from build123d import *

# Parameters (mm, degrees)
BOSS_EXTRUDE1_DEPTH       = 23.1
BOSS_EXTRUDE3_DEPTH       = 1
SKETCH8_R                 = 1.5
BOSS_EXTRUDE4_DEPTH       = 1
M8_TAPPED_HOLE1_D         = 6.8
M8_TAPPED_HOLE1_DEPTH     = 13.75
M8_TAPPED_HOLE1_TIP       = 2.042926105
F_4_0MM_DOWEL_HOLE1_D     = 4
F_4_0MM_DOWEL_HOLE1_DEPTH = 15
F_4_0MM_DOWEL_HOLE1_TIP   = 1.201721238
F_4_0MM_DOWEL_HOLE2_D     = 4
F_4_0MM_DOWEL_HOLE2_DEPTH = 15
F_4_0MM_DOWEL_HOLE2_TIP   = 1.201721238


with BuildPart() as part:
    # Sketch1 → Boss-Extrude1 (new body)
    with BuildSketch(Plane(origin=(0, 0, 0), x_dir=(1, 0, 0), z_dir=(0, 1, 0))):
        with BuildLine():
            Line((0, 7), (25, 7))
            ThreePointArc((25, 7), (32, 0), (25, -7))
            Line((25, -7), (0, -7))
            ThreePointArc((0, -7), (-7, 0), (0, 7))
        make_face()
    extrude(amount=BOSS_EXTRUDE1_DEPTH)

    # Sketch6 → Boss-Extrude3 (add)
    # profile 1 of 3: a face of its own
    with BuildSketch(Plane(origin=(0, 23.1, 0), x_dir=(1, 0, 0), z_dir=(0, 1, 0))):
        with BuildLine():
            Line((1.153846154, 4.5), (2.954927885, 4.5))
            add(Edge.make_bspline(
                [(2.954927885, 4.5), (3.075119358, 4.499599922), (3.305900301, 4.498831727), (3.636517282, 4.494548337), (3.936929817, 4.482271422), (4.206980832, 4.471706493), (4.446665374, 4.452441501), (4.656718407, 4.434028409), (4.836172486, 4.40992471), (4.944804675, 4.387539336), (4.993990385, 4.377403846)],
                knots=[0, 0, 0, 0, 1.410062039, 2.707475311, 3.878576406, 4.937260626, 5.877586885, 6.699081471, 7.410979367, 8, 8, 8, 8], degree=3))
            add(Edge.make_bspline(
                [(4.993990385, 4.377403846), (5.05983599, 4.361135021), (5.190122534, 4.328944429), (5.377708418, 4.260905455), (5.556459537, 4.182169278), (5.725633371, 4.08969114), (5.884382548, 3.982784563), (6.034343919, 3.863295106), (6.176197967, 3.731876576), (6.304207874, 3.585215555), (6.424908292, 3.431350245), (6.526707617, 3.264969156), (6.614461422, 3.090982371), (6.684328466, 2.907620439), (6.740586112, 2.716661597), (6.780253585, 2.51637612), (6.804042353, 2.30767647), (6.806464267, 2.165327562), (6.807692308, 2.093149038)],
                knots=[0, 0, 0, 0, 1.027469482, 2.033020251, 3.019912614, 3.986113645, 4.951240523, 5.91722682, 6.890402269, 7.87763091, 8.8651537, 9.85103654, 10.82876324, 11.815024772, 12.821070561, 13.842952187, 14.906261191, 16, 16, 16, 16], degree=3))
            add(Edge.make_bspline(
                [(6.807692308, 2.093149038), (6.803914884, 1.973230198), (6.796544152, 1.739237481), (6.727822457, 1.399652357), (6.615254263, 1.082879834), (6.460137234, 0.789318765), (6.26260144, 0.524691391), (6.025194834, 0.292258792), (5.747784976, 0.097756159), (5.489538163, -0.037122481), (5.261415936, -0.123504247), (5.073615988, -0.184283455), (4.868758046, -0.231242794), (4.6488049, -0.273311705), (4.412841215, -0.305073204), (4.161432542, -0.328335876), (3.894399581, -0.342874858), (3.710956259, -0.345040014), (3.616586538, -0.346153846)],
                knots=[0, 0, 0, 0, 1.260483769, 2.459530307, 3.627416485, 4.787058657, 5.939039949, 7.08810263, 8.267026773, 9.491475466, 10.141966685, 10.831826277, 11.566392101, 12.351337768, 13.187381173, 14.07005841, 15.007169909, 16, 16, 16, 16], degree=3))
            Line((3.616586538, -0.346153846), (6.923076923, -4.5))
            Line((6.923076923, -4.5), (5.924278846, -4.5))
            Line((5.924278846, -4.5), (2.617788462, -0.346153846))
            Line((2.617788462, -0.346153846), (1.961538462, -0.346153846))
            Line((1.961538462, -0.346153846), (1.961538462, -4.5))
            Line((1.961538462, -4.5), (1.153846154, -4.5))
            Line((1.153846154, -4.5), (1.153846154, 4.5))
        make_face()
        with BuildLine():
            Line((1.961538462, 3.576923077), (1.961538462, 0.576923077))
            Line((1.961538462, 0.576923077), (3.609375, 0.564302885))
            add(Edge.make_bspline(
                [(3.609375, 0.564302885), (3.686312243, 0.564268848), (3.835438533, 0.564202874), (4.051183099, 0.574472584), (4.252063387, 0.586155403), (4.437311035, 0.604025148), (4.6070088, 0.627055047), (4.761071863, 0.655862721), (4.89975171, 0.689425168), (5.061490809, 0.741372205), (5.242099033, 0.823673395), (5.43837993, 0.943413249), (5.605528798, 1.094019555), (5.746746158, 1.266237014), (5.860221839, 1.455587368), (5.940224265, 1.659800889), (5.990990545, 1.873722141), (5.996978233, 2.020751561), (6, 2.094951923)],
                knots=[0, 0, 0, 0, 1.146690395, 2.22261258, 3.21895312, 4.145990853, 4.996080663, 5.770904154, 6.481378293, 7.121626537, 8.300444488, 9.431385265, 10.535395872, 11.636531494, 12.74115979, 13.810798291, 14.895190096, 16, 16, 16, 16], degree=3))
            add(Edge.make_bspline(
                [(6, 2.094951923), (5.996908831, 2.167328827), (5.990783263, 2.310753441), (5.940772144, 2.520725781), (5.856199449, 2.718897939), (5.742227981, 2.904463757), (5.603373011, 3.072907078), (5.440555778, 3.217028329), (5.258228133, 3.335955524), (5.08781648, 3.411952502), (4.935499934, 3.458546411), (4.803252237, 3.491335118), (4.653822723, 3.517678038), (4.486485829, 3.53878448), (4.301955921, 3.556925765), (4.099299961, 3.569144625), (3.879862526, 3.576380275), (3.727770418, 3.576737932), (3.649038462, 3.576923077)],
                knots=[0, 0, 0, 0, 1.101028733, 2.181837193, 3.264309656, 4.369019818, 5.486613113, 6.575447106, 7.666700264, 8.788928104, 9.402425223, 10.0903467, 10.862060571, 11.710948788, 12.657782767, 13.684531032, 14.801375019, 16, 16, 16, 16], degree=3))
            Line((3.649038462, 3.576923077), (1.961538462, 3.576923077))
        make_face(mode=Mode.SUBTRACT)
    # profile 2 of 3: a face of its own
    with BuildSketch(Plane(origin=(0, 23.1, 0), x_dir=(1, 0, 0), z_dir=(0, 1, 0))):
        with BuildLine():
            Line((8.769230769, -4.5), (8.769230769, 4.5))
            Line((8.769230769, 4.5), (10.586538462, 4.5))
            add(Edge.make_bspline(
                [(10.586538462, 4.5), (10.744601574, 4.498861963), (11.049978685, 4.496663281), (11.491267835, 4.482722561), (11.899568939, 4.458061363), (12.273539148, 4.422139724), (12.614205122, 4.378031924), (12.920612971, 4.32274517), (13.194347053, 4.257461303), (13.362697043, 4.201801574), (13.442307692, 4.175480769)],
                knots=[0, 0, 0, 0, 1.314313732, 2.53924729, 3.670748893, 4.714932338, 5.66265055, 6.526160246, 7.303039223, 8, 8, 8, 8], degree=3))
            add(Edge.make_bspline(
                [(13.442307692, 4.175480769), (13.546437022, 4.135801812), (13.752334374, 4.057343684), (14.045495546, 3.909341767), (14.321475051, 3.741650933), (14.581752852, 3.554050144), (14.820383548, 3.341227533), (15.046689568, 3.112223599), (15.251413144, 2.858710724), (15.438891619, 2.585946469), (15.607926172, 2.297144049), (15.754855435, 1.99285377), (15.87687999, 1.674620949), (15.978176858, 1.343330568), (16.058010606, 0.998254168), (16.11247843, 0.638989941), (16.148403833, 0.26695774), (16.152014251, 0.014509119), (16.153846154, -0.113581731)],
                knots=[0, 0, 0, 0, 0.984719456, 1.947108742, 2.898477687, 3.838006223, 4.779231079, 5.722358779, 6.681677486, 7.655904652, 8.64651281, 9.637519902, 10.640069247, 11.656948941, 12.698408672, 13.768548281, 14.867775369, 16, 16, 16, 16], degree=3))
            add(Edge.make_bspline(
                [(16.153846154, -0.113581731), (16.152228809, -0.224824915), (16.149041662, -0.44404123), (16.120423421, -0.767117819), (16.078827169, -1.080609859), (16.014427804, -1.383024516), (15.936249912, -1.677011362), (15.83605638, -1.959437134), (15.72127939, -2.232892643), (15.587436845, -2.493680439), (15.440501855, -2.740751967), (15.282817372, -2.973660468), (15.114551584, -3.189082467), (14.934099957, -3.387670327), (14.7437944, -3.569124671), (14.542388979, -3.734961282), (14.329363991, -3.88193528), (14.105673561, -4.01582213), (13.864792086, -4.13261733), (13.602157001, -4.231437355), (13.316648258, -4.313328652), (13.008966655, -4.381653812), (12.678580569, -4.435852591), (12.325166085, -4.4721776), (11.949266198, -4.496742284), (11.691148087, -4.49889301), (11.558293269, -4.5)],
                knots=[0, 0, 0, 0, 1.105936401, 2.179363191, 3.223086493, 4.248585256, 5.251745608, 6.245858792, 7.225916811, 8.198733463, 9.158002045, 10.082870192, 10.993790845, 11.873723703, 12.748670949, 13.606408763, 14.465103618, 15.319838547, 16.196477973, 17.123216899, 18.106603292, 19.147568657, 20.255746949, 21.433717677, 22.679120308, 24, 24, 24, 24], degree=3))
            Line((11.558293269, -4.5), (8.769230769, -4.5))
        make_face()
        with BuildLine():
            Line((9.576923077, -3.576923077), (10.609975962, -3.576923077))
            add(Edge.make_bspline(
                [(10.609975962, -3.576923077), (10.758420343, -3.576285115), (11.043933254, -3.57505808), (11.45448239, -3.564290986), (11.829600838, -3.546697433), (12.169341862, -3.522075804), (12.473513639, -3.489499365), (12.742751853, -3.453178187), (12.976173945, -3.407927599), (13.117421069, -3.366910846), (13.182692308, -3.347956731)],
                knots=[0, 0, 0, 0, 1.375205317, 2.645023457, 3.804390687, 4.853969522, 5.800190428, 6.637939096, 7.370582563, 8, 8, 8, 8], degree=3))
            add(Edge.make_bspline(
                [(13.182692308, -3.347956731), (13.264845239, -3.319024152), (13.42718888, -3.26185005), (13.660883099, -3.157558921), (13.878829682, -3.03402217), (14.08482689, -2.896702037), (14.275952576, -2.740755175), (14.454471732, -2.569572632), (14.620024935, -2.382283211), (14.770901727, -2.179119367), (14.90592308, -1.961345606), (15.022849099, -1.731102891), (15.125324466, -1.490913951), (15.205755133, -1.2370904), (15.268795206, -0.971901392), (15.313447261, -0.695328273), (15.341256552, -0.407422691), (15.344500276, -0.211602943), (15.346153846, -0.111778846)],
                knots=[0, 0, 0, 0, 0.998632004, 1.973411704, 2.929992603, 3.868527914, 4.809262121, 5.754881198, 6.702106254, 7.672490631, 8.653608572, 9.636854334, 10.631411391, 11.644891563, 12.686317036, 13.754757253, 14.855430412, 16, 16, 16, 16], degree=3))
            add(Edge.make_bspline(
                [(15.346153846, -0.111778846), (15.344833964, -0.006521325), (15.342241045, 0.200258006), (15.309649961, 0.503662651), (15.262023104, 0.795470038), (15.193150768, 1.075699683), (15.105385651, 1.344898303), (14.995856573, 1.601577044), (14.870713837, 1.848446706), (14.721819543, 2.079809361), (14.558750874, 2.298620213), (14.377779184, 2.49907571), (14.181779657, 2.681632483), (13.972890044, 2.849133572), (13.745223217, 2.994840167), (13.504142298, 3.125177347), (13.246110572, 3.235789639), (13.066592211, 3.294621001), (12.975360577, 3.324519231)],
                knots=[0, 0, 0, 0, 1.122418816, 2.205001699, 3.251619955, 4.274784885, 5.280384055, 6.268708349, 7.249350384, 8.229342522, 9.199999885, 10.157847722, 11.105861043, 12.055065948, 13.010012805, 13.98527497, 14.976112212, 16, 16, 16, 16], degree=3))
            add(Edge.make_bspline(
                [(12.975360577, 3.324519231), (12.899886201, 3.345390045), (12.739406968, 3.389767123), (12.477534061, 3.438175224), (12.182809391, 3.480872507), (11.853924445, 3.517021751), (11.491254122, 3.542960578), (11.094519496, 3.562429672), (10.663549084, 3.575561013), (10.364793997, 3.576457689), (10.209735577, 3.576923077)],
                knots=[0, 0, 0, 0, 0.674548936, 1.434276114, 2.292660221, 3.240891867, 4.284742987, 5.42552168, 6.663806718, 8, 8, 8, 8], degree=3))
            Line((10.209735577, 3.576923077), (9.576923077, 3.576923077))
            Line((9.576923077, 3.576923077), (9.576923077, -3.576923077))
        make_face(mode=Mode.SUBTRACT)
    # profile 3 of 3: a face of its own
    with BuildSketch(Plane(origin=(0, 23.1, 0), x_dir=(1, 0, 0), z_dir=(0, 1, 0))):
        Polygon((17.307692308, 4.5), (18.173076923, 4.5), (21.173076923, -2.592548077), (24.173076923, 4.5), (25.038461538, 4.5), (21.230769231, -4.5), (21.115384615, -4.5), align=None)
    extrude(amount=BOSS_EXTRUDE3_DEPTH)

    # Sketch8 → Boss-Extrude4 (add)
    with BuildSketch(Plane(origin=(0, 23.1, 0), x_dir=(1, 0, 0), z_dir=(0, 1, 0))):
        with Locations(Location((-4, 0, 0), (0, 0, 270))):
            Circle(SKETCH8_R)
    extrude(amount=BOSS_EXTRUDE4_DEPTH)

    # M8 Tapped Hole1
    with Locations(Plane(origin=(12.5, 0, 0), x_dir=(0, 0, -1), z_dir=(0, -1, 0))):
        with Locations((0, 0)):
            Hole(M8_TAPPED_HOLE1_D / 2, depth=M8_TAPPED_HOLE1_DEPTH)
            with Locations((0, 0, -(M8_TAPPED_HOLE1_DEPTH + M8_TAPPED_HOLE1_TIP / 2))):  # 118° drill point
                Cone(0, M8_TAPPED_HOLE1_D / 2, M8_TAPPED_HOLE1_TIP, mode=Mode.SUBTRACT)

    # Ø4.0mm Dowel Hole1
    with Locations(Plane(origin=(2.5, 0, 0), x_dir=(0, 0, -1), z_dir=(0, -1, 0))):
        with Locations((0, 0)):
            Hole(F_4_0MM_DOWEL_HOLE1_D / 2, depth=F_4_0MM_DOWEL_HOLE1_DEPTH)
            with Locations((0, 0, -(F_4_0MM_DOWEL_HOLE1_DEPTH + F_4_0MM_DOWEL_HOLE1_TIP / 2))):  # 118° drill point
                Cone(0, F_4_0MM_DOWEL_HOLE1_D / 2, F_4_0MM_DOWEL_HOLE1_TIP, mode=Mode.SUBTRACT)

    # Ø4.0mm Dowel Hole2
    with Locations(Plane(origin=(22.5, 0, 0), x_dir=(0, 0, -1), z_dir=(0, -1, 0))):
        with Locations((0, 0)):
            Hole(F_4_0MM_DOWEL_HOLE2_D / 2, depth=F_4_0MM_DOWEL_HOLE2_DEPTH)
            with Locations((0, 0, -(F_4_0MM_DOWEL_HOLE2_DEPTH + F_4_0MM_DOWEL_HOLE2_TIP / 2))):  # 118° drill point
                Cone(0, F_4_0MM_DOWEL_HOLE2_D / 2, F_4_0MM_DOWEL_HOLE2_TIP, mode=Mode.SUBTRACT)


solid = part.part
Verification items for the finished model (mm, model axes). A direction names the side the tool comes from. Coordinates: 2 decimals unless noted, no trailing zeros. Write each loop counter-clockwise with the first axis right and the second up, starting at its lowest first coordinate (ties: lowest second). Pieces come first, ordered by that corner, then holes. Notation, with made-up numbers: (71.25, 11.25) - (111.25, 11.25) arc R25 ccw to (111.25, 29.25) - close; hole circle Ø10 at (-7.5, 61). An arc over 180 degrees is marked (long way). Answer as a JSON object with one key per item and string values.
(1) Mould release check, pull along Z, two halves, no side actions. Record for faces 1 (the flat face through (5.247, 23.593, 2.394)), 2 (the cylindrical face through (32, 11, 0)), 3 (the flat face through (17.7, 23.6, -4.5)): pulls with the +Z half, pulls with the -Z half, needs draft (parallel to the pull), parting line crosses it, or undercut.
Report:
{"face 1": "undercut", "face 2": "parting line crosses it", "face 3": "pulls with the -Z half"}
(2) Cross-section at C-C on y = 19.75. Record the cut outline in (x, z), plus the area to 3 significant figures.
Report:
{"outline": "(0, -7) - (25, -7) arc R7 ccw to (25, 7) - (0, 7) arc R7 ccw to start", "area": "504 mm^2"}
(3) Thickness scan on line 1 along X through (y, z) = (4, 0); line 2 along Z through (x, y) = (22.5, 3); line 3 along X through (y, z) = (5, -1). Record the ranges inside material, lowest first.
Report:
{"line 1": "-7 to 0.5, 4.5 to 9.1, 15.9 to 20.5, 24.5 to 32", "line 2": "-7 to -2, 2 to 7", "line 3": "-6.93 to 0.77, 4.23 to 9.25, 15.75 to 20.77, 24.23 to 31.93"}
(4) Gauge pin test, flat ends, axial feed: pin 1 Ø1 at (x, y) = (18, 24) entering from -Z; pin 2 Ø1.5 at (y, z) = (9, 5.5) entering from -X; pin 3 Ø0.5 at (x, y) = (10, 23.5) entering from +Z. Record the tip position at first contact, or that the pin passes through.
Report:
{"pin 1": "z = -4.5", "pin 2": "x = -5.14", "pin 3": "z = 4.5"}
(5) Tool access check on faces 4 (the cylindrical face through (9.18, 6.97, -0.74)), 5 (the flat face through (1.962, 23.6, 2.4)), 6 (the flat face through (10.2, 23.6, 4.5)), 7 (the cylindrical face through (-2.513, 23.593, -0.195)). Record the directions out of +Z, -Z, +X, -X, +Y, -Y that give a thin tool (end or side, any length) a straight path to the whole face; none if there is none.
Report:
{"face 4": "-Y", "face 5": "+Z, +Y", "face 6": "+Z, +X, -X, +Y", "face 7": "+Y"}
(6) Cross-section at A-A on y = 4. Record the cut outline in (x, z), plus the area to 3 significant figures.
Report:
{"outline": "(0, -7) - (25, -7) arc R7 ccw to (25, 7) - (0, 7) arc R7 ccw to start; hole circle Ø4 at (2.5, 0); hole circle Ø6.8 at (12.5, 0); hole circle Ø4 at (22.5, 0)", "area": "442 mm^2"}
(7) Cross-section at D-D on z = -5. Record the cut outline in (x, y).
Report:
{"outline": "(-4.9, 0) - (29.9, 0) - (29.9, 23.1) - (-4.9, 23.1) - close"}
(8) Cross-section at B-B on x = -3.5. Record the cut outline in (y, z).
Report:
{"outline": "(0, -6.06) - (23.1, -6.06) - (23.1, -1.41) - (24.1, -1.41) - (24.1, 1.41) - (23.1, 1.41) - (23.1, 6.06) - (0, 6.06) - close"}
